Source: CAD feature listing. Evaluate the final solid. Frame: model axes, mm. A direction names the side the tool comes from. Round coordinates to 2 decimals unless told otherwise and drop trailing zeros. Loops run counter-clockwise (first coordinate to the right, second up) from the corner with the lowest first, then second, coordinate; pieces in that order, holes last. Notation, with made-up numbers: M -7.75,53.25 L -3.75,53.25 A24 ccw -3.75,91.25 Z; hole C 57,81.5 d2. An arc over 180 degrees is marked long. Answer as CSV lines item,"result". Start each with the question number.
```python
from build123d import *

# Parameters (mm, degrees)
F0_W     = 80
F0_H     = 50
F1_DEPTH = 9.525
F3_DEPTH = 25
F4_R     = 4.7625
F5_DEPTH = 9.526


with BuildPart() as f1:
    # F0 (on Top) → F1 (new body)
    with BuildSketch(Plane.XY):
        Rectangle(F0_W, F0_H)
    extrude(amount=F1_DEPTH)

    # F2 (on face) → F3 (cut)
    with BuildSketch(Plane.XY.offset(9.525)):
        with BuildLine():
            ThreePointArc((-29.3, 18.933095), (-32, 21.633095), (-34.7, 18.933095))
            Line((-34.7, 18.933095), (-34.7, 8.933095))
            ThreePointArc((-34.7, 8.933095), (-32, 6.233095), (-29.3, 8.933095))
            Line((-29.3, 8.933095), (-29.3, 18.933095))
        make_face()
        with BuildLine():
            ThreePointArc((-34.7, -18.933095), (-32, -21.633095), (-29.3, -18.933095))
            Line((-29.3, -18.933095), (-29.3, -8.933095))
            ThreePointArc((-29.3, -8.933095), (-32, -6.233095), (-34.7, -8.933095))
            Line((-34.7, -8.933095), (-34.7, -18.933095))
        make_face()
        with BuildLine():
            ThreePointArc((29.3, -18.933095), (32, -21.633095), (34.7, -18.933095))
            Line((34.7, -18.933095), (34.7, -8.933095))
            ThreePointArc((34.7, -8.933095), (32, -6.233095), (29.3, -8.933095))
            Line((29.3, -8.933095), (29.3, -18.933095))
        make_face()
        with BuildLine():
            ThreePointArc((34.7, 18.933095), (32, 21.633095), (29.3, 18.933095))
            Line((29.3, 18.933095), (29.3, 8.933095))
            ThreePointArc((29.3, 8.933095), (32, 6.233095), (34.7, 8.933095))
            Line((34.7, 8.933095), (34.7, 18.933095))
        make_face()
    extrude(amount=-F3_DEPTH, mode=Mode.SUBTRACT)

    # F4 (on face) → F5 (cut, through all)
    with BuildSketch(Plane.XY.offset(9.525)):
        with Locations((0, 4.68)):
            Circle(F4_R)
    extrude(amount=-F5_DEPTH, mode=Mode.SUBTRACT)


solid = f1.part
```
1) Section A-A, the plane y = 14.5. Return loops of the section in (x, z) (3 decimals), and give its area (3 significant figures).
2) Section D-D, the plane y = 4.68. Return loops of the section in (x, z) (1 decimal), and give its area (3 significant figures).
3) Access query for faces 4 (the cylindrical face through (-32.059, 6.234, 4.829)), 5 (the flat face through (-1, -5, 9.525)). Directions: +Z, -Z, +X, -X, +Y, -Y. A direction counts if a zero-diameter tool reaches every point of the face in a straight line with its end or side. Return the directions, or none.
4) Section B-B, the plane x = 32. Return loops of the section in (y, z) (3 decimals), and give its area (3 significant figures).
5) Ray query, line 1 along X through (y, z) = (14, 3.5); line 2 along X through (y, z) = (7.5, 1.25); line 3 along Y through (x, z) = (-31.5, 1.5). Return the intervals inside material, ascending.
6) Section C-C, the plane x = 0. Return loops of the section in (y, z) (1 decimal).
7) Mould query, pull axis Y, two halves, no side actions, for faces 1 (the flat face through (-1, 25, 5)), 2 (the flat face through (-29.3, 14, 5)), 3 (the flat face through (-40, 0, 5)). Classes: pulls with the +Y half, pulls with the -Y half, needs draft (parallel to the pull), parting line crosses it, or undercut.
Findings below:
1,outline,"M -40,0 L -34.7,0 L -34.7,9.525 L -40,9.525 Z; M -29.3,0 L 29.3,0 L 29.3,9.525 L -29.3,9.525 Z; M 34.7,0 L 40,0 L 40,9.525 L 34.7,9.525 Z"
1,area,"659 mm²"
2,outline,"M -40,0 L -4.8,0 L -4.8,9.5 L -40,9.5 Z; M 4.8,0 L 40,0 L 40,9.5 L 4.8,9.5 Z"
2,area,"671 mm²"
3,face 4,"+Z, -Z"
3,face 5,"+Z, +X, -X, +Y, -Y"
4,outline,"M -25,0 L -21.633,0 L -21.633,9.525 L -25,9.525 Z; M -6.233,0 L 6.233,0 L 6.233,9.525 L -6.233,9.525 Z; M 21.633,0 L 25,0 L 25,9.525 L 21.633,9.525 Z"
4,area,"183 mm²"
5,line 1,"-40 to -34.7, -29.3 to 29.3, 34.7 to 40"
5,line 2,"-40 to -34.29, -29.71 to -3.84, 3.84 to 29.71, 34.29 to 40"
5,line 3,"-25 to -21.59, -6.28 to 6.28, 21.59 to 25"
6,outline,"M -25,0 L -0.1,0 L -0.1,9.5 L -25,9.5 Z; M 9.4,0 L 25,0 L 25,9.5 L 9.4,9.5 Z"
7,face 1,"pulls with the +Y half"
7,face 2,"undercut"
7,face 3,"needs draft"
